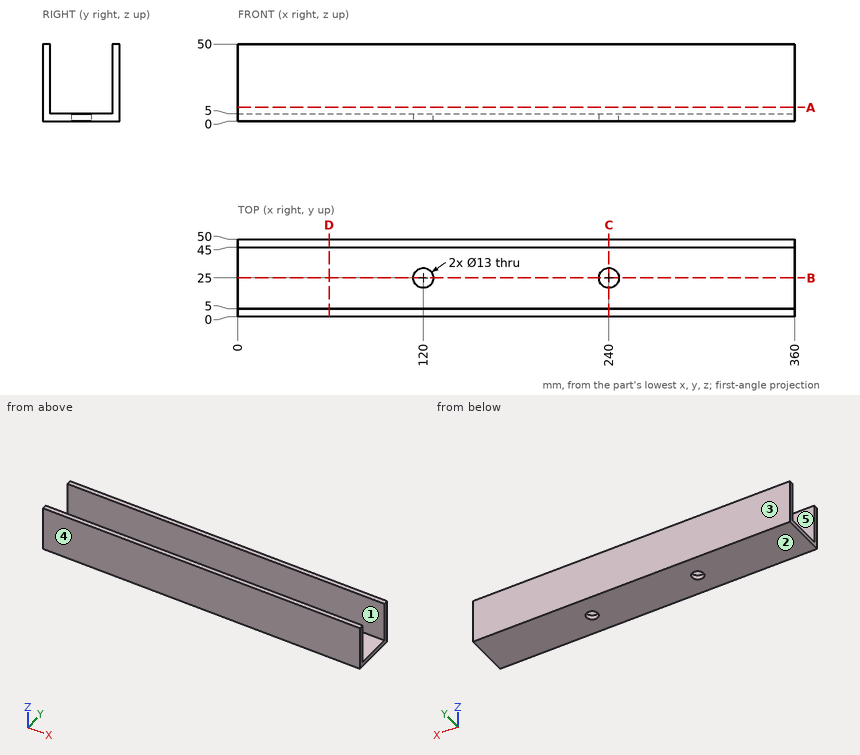
Job drawing, mm, ordinate dimensions from the low corner. One solid piece. A direction names the side the tool comes from. Round coordinates to 2 decimals unless told otherwise and drop trailing zeros. Loops run counter-clockwise (first coordinate to the right, second up) from the corner with the lowest first, then second, coordinate; pieces in that order, holes last. Notation, with made-up numbers: (-8.75, -17) -> (5.25, -17) arc R27 cw to (5.25, 11) -> close; hole circle Ø6 at (-9, 83). An arc over 180 degrees is marked (long way). Use a Markdown table: item, result.
1) Cut at A-A, the plane z = 9. List the corners of the cut face in (x, y), and give its area (3 significant figures).
The answers:
| item | result |
|---|---|
| outline | (0, 0) -> (360, 0) -> (360, 5) -> (0, 5) -> close; (0, 45) -> (360, 45) -> (360, 50) -> (0, 50) -> close |
| area | 3,600 mm2 |
2) Drop a flat-ended pin along its axis: pin 1 Ø20 at (x, y) = (182, 26) entering from +Z. Give the stop position or say it passes through.
The answers:
| item | result |
|---|---|
| pin 1 | stops at z = 5 |
3) Cut at D-D, the plane x = 59. List the corners of the cut face in (y, z).
The answers:
| item | result |
|---|---|
| outline | (0, 0) -> (50, 0) -> (50, 50) -> (45, 50) -> (45, 5) -> (5, 5) -> (5, 50) -> (0, 50) -> close |
4) Cut at B-B, the plane y = 25. List the corners of the cut face in (x, z), and give its area (3 significant figures).
The answers:
| item | result |
|---|---|
| outline | (0, 0) -> (113.5, 0) -> (113.5, 5) -> (0, 5) -> close; (126.5, 0) -> (233.5, 0) -> (233.5, 5) -> (126.5, 5) -> close; (246.5, 0) -> (360, 0) -> (360, 5) -> (246.5, 5) -> close |
| area | 1,670 mm2 |
5) Cut at C-C, the plane x = 240. List the corners of the cut face in (y, z).
The answers:
| item | result |
|---|---|
| outline | (0, 0) -> (18.5, 0) -> (18.5, 5) -> (5, 5) -> (5, 50) -> (0, 50) -> close; (31.5, 0) -> (50, 0) -> (50, 50) -> (45, 50) -> (45, 5) -> (31.5, 5) -> close |
6) Pull direction Y, two halves, no side cores. Call the marked faces 3, 4 and 5: pulls with the +Y half, pulls with the -Y half, needs draft (parallel to the pull), parting line crosses it, or undercut.
The answers:
| item | result |
|---|---|
| face 3 | pulls with the +Y half |
| face 4 | pulls with the -Y half |
| face 5 | undercut |
7) Tool access for the marked faces 1 and 2: list every direction of +Z, -Z, +X, -X, +Y, -Y with a clear straight run to the whole face (end or side of a thin tool).
The answers:
| item | result |
|---|---|
| face 1 | +Z, +X, -X |
| face 2 | -Z, +X, -X, +Y, -Y |
8) Probe line 1 (X direction, y = 25, z = 2.95); line 2 (Y direction, x = 223.5, z = 24); line 3 (Y direction, x = 240, z = 3.85). List the from-to ranges inside material, lowest first. Write a range as [from, to].
The answers:
| item | result |
|---|---|
| line 1 | x = [0, 113.5], [126.5, 233.5], [246.5, 360] |
| line 2 | y = [0, 5], [45, 50] |
| line 3 | y = [0, 18.5], [31.5, 50] |
